Source: three-view drawing plus pictorial views. Frame: mm from the lowest corner of the part. A direction names the side the tool comes from. Round coordinates to 2 decimals unless told otherwise and drop trailing zeros. Loops run counter-clockwise (first coordinate to the right, second up) from the corner with the lowest first, then second, coordinate; pieces in that order, holes last. Notation, with made-up numbers: (73.25, -17.5) -> (81.25, -17.5) arc R6 ccw to (81.25, -10.5) -> close; hole circle Ø10 at (-38.5, 19.5). An arc over 180 degrees is marked (long way). Answer in a Markdown table with one row per item.
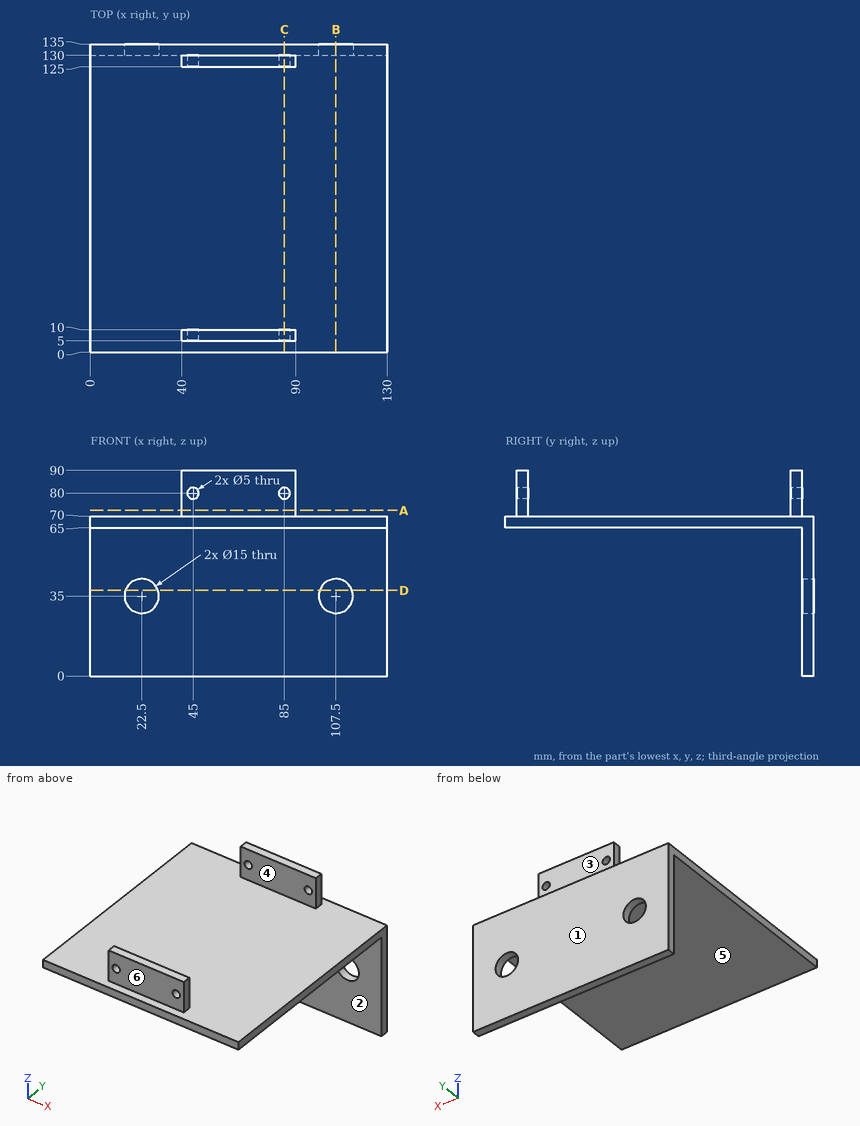
Item 1: Line query: probe 1 along Z at (x, y) = (85, 8.85); probe 2 along Z at (x, y) = (22, 133); probe 3 along Y at (x, z) = (93.5, 43). Output: solid intervals per line, ascending. Write a range as [from, to].
Answer:
| item | result |
|---|---|
| probe 1 | z = [65, 77.5], [82.5, 90] |
| probe 2 | z = [0, 27.52], [42.48, 70] |
| probe 3 | y = [130, 135] |
Item 2: Reachability of the marked faces 1, 2 and 3 from +Z, -Z, +X, -X, +Y, -Y: full face, straight path, thin tool, end or side. Return the list, or none.
Answer:
| item | result |
|---|---|
| face 1 | +Z, -Z, +X, -X, +Y |
| face 2 | -Z, +X, -X, -Y |
| face 3 | +Z, +X, -X, +Y |
Item 3: Cut plane A-A (z = 72.5). Output: boundary loops of the cut face in (x, y).
Answer:
| item | result |
|---|---|
| outline | (40, 5) -> (90, 5) -> (90, 10) -> (40, 10) -> close; (40, 125) -> (90, 125) -> (90, 130) -> (40, 130) -> close |
Item 4: Cut plane D-D (z = 37.5). Output: boundary loops of the cut face in (x, y), then the cut area to 3 significant figures.
Answer:
| item | result |
|---|---|
| outline | (0, 130) -> (15.43, 130) -> (15.43, 135) -> (0, 135) -> close; (29.57, 130) -> (100.43, 130) -> (100.43, 135) -> (29.57, 135) -> close; (114.57, 130) -> (130, 130) -> (130, 135) -> (114.57, 135) -> close |
| area | 509 mm² |
Item 5: Draft query along Y for the marked faces 4, 5 and 6. Return one class per face: pulls with the +Y half, pulls with the -Y half, needs draft (parallel to the pull), parting line crosses it, or undercut.
Answer:
| item | result |
|---|---|
| face 4 | undercut |
| face 5 | needs draft |
| face 6 | pulls with the -Y half |
Item 6: Pin query (flat end, axial travel): pin 1 Ø5 at (x, y) = (27.5, 61.5) entering from -Z; pin 2 Ø19.5 at (x, z) = (22.5, 35) entering from -Y; pin 3 Ø10 at (x, z) = (72.5, 80.5) entering from -Y; pin 4 Ø4.5 at (x, z) = (45, 80) entering from +Y. Return the tip coordinate at first contact, or that it passes through.
Answer:
| item | result |
|---|---|
| pin 1 | stops at z = 65 |
| pin 2 | stops at y = 130 |
| pin 3 | stops at y = 5 |
| pin 4 | passes through |
Item 7: Cut plane B-B (x = 107.5). Output: boundary loops of the cut face in (y, z), then the cut area to 3 significant figures.
Answer:
| item | result |
|---|---|
| outline | (0, 65) -> (130, 65) -> (130, 42.5) -> (135, 42.5) -> (135, 70) -> (0, 70) -> close; (130, 0) -> (135, 0) -> (135, 27.5) -> (130, 27.5) -> close |
| area | 925 mm² |
Item 8: Cut plane C-C (x = 85). Output: boundary loops of the cut face in (y, z), then the cut area to 3 significant figures.
Answer:
| item | result |
|---|---|
| outline | (0, 65) -> (130, 65) -> (130, 0) -> (135, 0) -> (135, 70) -> (130, 70) -> (130, 77.5) -> (125, 77.5) -> (125, 70) -> (10, 70) -> (10, 77.5) -> (5, 77.5) -> (5, 70) -> (0, 70) -> close; (5, 82.5) -> (10, 82.5) -> (10, 90) -> (5, 90) -> close; (125, 82.5) -> (130, 82.5) -> (130, 90) -> (125, 90) -> close |
| area | 1,150 mm² |
